Work out the finished part from the listing and answer in its coordinate system (mm). A direction names the side the tool comes from. Give positions to 0.01 mm unless a question says otherwise; leave off trailing zeros. Loops run counter-clockwise (first coordinate to the right, second up) from the corner with the lowest first, then second, coordinate; pieces in that order, holes last. Notation, with made-up numbers: M 27.5,81 L 73.5,81 A35 ccw 73.5,116 Z; hole C 32.25,87.5 d2. An arc over 180 degrees is marked long. Write item = value, one per line. Start each with the question number.
1. Section C-C on z = 21 is taken. Give the number of separate pieces and of enclosed holes in the cut face, plus the area to 3 significant figures.
2. Section B-B on y = 10 is taken. Determine the outline of the cut face in (x, z).
3. Section D-D on x = 82 is taken. Determine the outline of the cut face in (y, z).
4. For faces 1 (the face through (41.498, 64.255, 0.74)), 2 (the face through (66, -3, 16)), 3 (the face through (124.169, 10.526, 2.24)), 4 (the face through (0.9, 0.86, 18.21)), 5 (the face through (131, 41, 6)), determine the directions among +Z, -Z, +X, -X, +Y, -Y from which every point of the face is accessible in a straight line to the end or side of a thin tool.
5. The mould has two halves that part along Y. Classify faces 6 (the face through (132, 101, 17)), 7 (the face through (46.169, 17.026, 2.24)), 8 (the face through (-3, 49, 16)), 9 (the face through (105, 98, 3)): released by +Y, released by -Y, zero draft, split by the parting line, or undercut.
6. Section A-A on x = 44.5 is taken. Determine the outline of the cut face in (y, z), plus the area to 3 significant figures.
7. Consider L1, parallel to Y at x = 105.5, z = 23.25 (3 decimals); L2, parallel to Y at x = 77, z = 18.5; L3, parallel to X at y = 72, z = 22.5. Determine where each line is inside the solid, lowest interval first. Write a range as [from, to].
8. Flat-ended cylindrical pins translate along their axes: pin 1 Ø4 at (x, y) = (102, 65.5) entering from -Z; pin 2 Ø1.5 at (y, z) = (-1, 9.5) entering from -X; pin 3 Ø4 at (x, y) = (102, 16.5) entering from +Z. Find the tip coordinate at first contact, or state that the pin passes through.
```python
from build123d import *

# Parameters (mm, degrees)
ESQUISSE1_W                = 130
ESQUISSE1_H                = 100
ESQUISSE1_R                = 1.75
BOSS_EXTRU_1_DEPTH         = 3
ESQUISSE2_R                = 3.25
ENL_V_MAT_EXTRU_1_DEPTH    = 1.5
ESQUISSE3_W                = 136
ESQUISSE3_H                = 106
ESQUISSE3_W_2              = 130
ESQUISSE3_H_2              = 100
BOSS_EXTRU_2_DEPTH         = 33
CONG_1_R                   = 3
CONG_2_R                   = 5
ESQUISSE4_W                = 20
ESQUISSE4_H                = 54
ENL_V_MAT_EXTRU_2_DEPTH    = 3
ESQUISSE5_W                = 15
ESQUISSE5_H                = 8
ENL_V_MAT_EXTRU_3_DEPTH    = 3
ESQUISSE6_R                = 2.375
BOSS_EXTRU_3_DEPTH         = 30
R_P_TITION_LIN_AIRE1_COUNT = 2
R_P_TITION_LIN_AIRE1_PITCH = 80


with BuildPart() as part:
    # Esquisse1 → Boss.-Extru.1 (new body)
    with BuildSketch(Plane.XY):
        with Locations((65, 50)):
            Rectangle(ESQUISSE1_W, ESQUISSE1_H)
        with Locations((122.5, 10)):
            Circle(ESQUISSE1_R, mode=Mode.SUBTRACT)
        with Locations((122.5, 94)):
            Circle(ESQUISSE1_R, mode=Mode.SUBTRACT)
        with Locations((7.5, 94)):
            Circle(ESQUISSE1_R, mode=Mode.SUBTRACT)
        with Locations((7.5, 10)):
            Circle(ESQUISSE1_R, mode=Mode.SUBTRACT)
        with Locations((44.5, 65.5)):
            Circle(ESQUISSE1_R, mode=Mode.SUBTRACT)
        with Locations((102, 65.5)):
            Circle(ESQUISSE1_R, mode=Mode.SUBTRACT)
        with Locations((102, 16.5)):
            Circle(ESQUISSE1_R, mode=Mode.SUBTRACT)
        with Locations((44.5, 16.5)):
            Circle(ESQUISSE1_R, mode=Mode.SUBTRACT)
    extrude(amount=BOSS_EXTRU_1_DEPTH)

    # Esquisse2 → Enlèv. mat.-Extru.1 (cut)
    with BuildSketch(Plane(origin=(0, 0, 0), x_dir=(-1, 0, 0), z_dir=(0, 0, -1))):
        with Locations((-102, 16.5)):
            Circle(ESQUISSE2_R)
        with Locations((-122.5, 10)):
            Circle(ESQUISSE2_R)
        with Locations((-122.5, 94)):
            Circle(ESQUISSE2_R)
        with Locations((-102, 65.5)):
            Circle(ESQUISSE2_R)
        with Locations((-44.5, 65.5)):
            Circle(ESQUISSE2_R)
        with Locations((-44.5, 16.5)):
            Circle(ESQUISSE2_R)
        with Locations((-7.5, 10)):
            Circle(ESQUISSE2_R)
        with Locations((-7.5, 94)):
            Circle(ESQUISSE2_R)
    extrude(amount=-ENL_V_MAT_EXTRU_1_DEPTH, mode=Mode.SUBTRACT)

    # Esquisse3 → Boss.-Extru.2 (add)
    with BuildSketch(Plane(origin=(0, 0, 0), x_dir=(-1, 0, 0), z_dir=(0, 0, -1))):
        with Locations((-65, 50)):
            Rectangle(ESQUISSE3_W, ESQUISSE3_H)
        with Locations((-65, 50)):
            Rectangle(ESQUISSE3_W_2, ESQUISSE3_H_2, mode=Mode.SUBTRACT)
    extrude(amount=-BOSS_EXTRU_2_DEPTH)

    # Congé1
    cong_1_edges = [part.edges().sort_by_distance(p)[0] for p in [
        (130, 0, 18),
        (0, 100, 18),
        (0, 0, 18),
        (130, 100, 18),
    ]]
    fillet(cong_1_edges, radius=CONG_1_R)

    # Congé2
    cong_2_edges = [part.edges().sort_by_distance(p)[0] for p in [
        (-3, 103, 16.5),
        (-3, -3, 16.5),
        (133, -3, 16.5),
        (133, 103, 16.5),
    ]]
    fillet(cong_2_edges, radius=CONG_2_R)

    # Esquisse4 → Enlèv. mat.-Extru.2 (cut)
    with BuildSketch(Plane.ZY.offset(-130)):
        with Locations((16, 41)):
            Rectangle(ESQUISSE4_W, ESQUISSE4_H)
    extrude(amount=-ENL_V_MAT_EXTRU_2_DEPTH, mode=Mode.SUBTRACT)

    # Esquisse5 → Enlèv. mat.-Extru.3 (cut)
    with BuildSketch(Plane(origin=(0, 0, 0), x_dir=(1, 0, 0), z_dir=(0, 1, 0))):
        with Locations((49.5, -9)):
            Rectangle(ESQUISSE5_W, ESQUISSE5_H)
    extrude(amount=-ENL_V_MAT_EXTRU_3_DEPTH, mode=Mode.SUBTRACT)

    # Esquisse6 → Boss.-Extru.3 (add)
    with BuildSketch(Plane.XY.offset(3)):
        with BuildLine():
            Line((20, 97.525), (20, 100))
            Line((20, 100), (31, 100))
            Line((31, 100), (31, 97.525))
            ThreePointArc((31, 97.525), (25.5, 92.025), (20, 97.525))
        make_face()
        with Locations((25.5, 97.525)):
            Circle(ESQUISSE6_R, mode=Mode.SUBTRACT)
        with BuildLine():
            Line((31, 2.475), (31, 0))
            Line((31, 0), (20, 0))
            Line((20, 0), (20, 2.475))
            ThreePointArc((20, 2.475), (25.5, 7.975), (31, 2.475))
        make_face()
        with Locations((25.5, 2.475)):
            Circle(ESQUISSE6_R, mode=Mode.SUBTRACT)
    boss_extru_3 = extrude(amount=BOSS_EXTRU_3_DEPTH)

    # Répétition linéaire1: Boss.-Extru.3 ×2
    with Locations(*[(i * R_P_TITION_LIN_AIRE1_PITCH, 0, 0) for i in range(1, R_P_TITION_LIN_AIRE1_COUNT)]):
        add(boss_extru_3)


solid = part.part
```
Verdict:
q1.separate_pieces = 1
q1.enclosed_holes = 4
q1.area = 1,470 mm2
q2.outline = M -3,0 L 4.25,0 L 4.25,1.5 L 5.75,1.5 L 5.75,3 L 0,3 L 0,33 L -3,33 Z; M 9.25,1.5 L 10.75,1.5 L 10.75,0 L 119.25,0 L 119.25,1.5 L 120.75,1.5 L 120.75,3 L 9.25,3 Z; M 124.25,1.5 L 125.75,1.5 L 125.75,0 L 133,0 L 133,33 L 130,33 L 130,3 L 124.25,3 Z
q3.outline = M -3,0 L 103,0 L 103,33 L 100,33 L 100,3 L 0,3 L 0,33 L -3,33 Z
q4.face_1 = -Z
q4.face_2 = +Z, -Z, +X, -X, -Y
q4.face_3 = +Z, -Z
q4.face_4 = +Z
q4.face_5 = +X
q5.face_6 = released by +Y
q5.face_7 = undercut
q5.face_8 = zero draft
q5.face_9 = undercut
q6.outline = M -3,0 L 13.25,0 L 13.25,1.5 L 14.75,1.5 L 14.75,3 L 0,3 L 0,5 L -3,5 Z; M -3,13 L 0,13 L 0,33 L -3,33 Z; M 18.25,1.5 L 19.75,1.5 L 19.75,0 L 62.25,0 L 62.25,1.5 L 63.75,1.5 L 63.75,3 L 18.25,3 Z; M 67.25,1.5 L 68.75,1.5 L 68.75,0 L 103,0 L 103,33 L 100,33 L 100,3 L 67.25,3 Z
q6.area = 444 mm2
q7.L1 = [-3, 0.1], [4.85, 7.975], [92.025, 95.15], [99.9, 103]
q7.L2 = [-3, 0], [100, 103]
q7.L3 = [-3, 0], [130, 133]
q8.pin_1 = 1.5
q8.pin_2 = -2.47
q8.pin_3 = 3
